Part model, mm, in its own coordinate system. A direction names the side the tool comes from. Give positions to 0.01 mm unless a question says otherwise; leave off trailing zeros. Order: outer loops, then holes, each group sorted by start corner. A loop starts at its lowest first (then second) coordinate and runs counter-clockwise, first axis right, second up.
Autodesk Inventor part; units mm, degrees
ref_plane "YZ Plane" through (0, 0, 0) normal (1, 0, 0) x (0, 1, 0)
ref_plane "XZ Plane" through (0, 0, 0) normal (0, 1, 0) x (-1, 0, 0)
ref_plane "XY Plane" through (0, 0, 0) normal (0, 0, 1) x (1, 0, 0)
sketch "Sketch2" plane through (0, 0, 0) normal (0, 0, 1) x (1, 0, 0)
  circle A0 centre (138.7343, -109.7729) radius 5.25
  circle A1 centre (116.8119, -56.8475) radius 5.25
  circle A2 centre (26.4627, 2.4988) radius 5.25
  circle A3 centre (79.388, -19.4236) radius 5.25
  line L0 (116.6514, -65.861) -> (120.8614, -63.1603)
  arc A4 (120.8614, -63.1603) -> (112.4329, -50.7586) centre (116.8119, -56.8475) ccw
  line L1 (112.4329, -50.7586) -> (108.3722, -53.679)
  arc A5 (108.3722, -53.679) -> (82.5566, -27.8633) centre (0, -136.2355) ccw
  line L2 (82.5566, -27.8633) -> (85.4769, -23.8026)
  arc A6 (85.4769, -23.8026) -> (73.0752, -15.3741) centre (79.388, -19.4236) ccw
  line L3 (73.0752, -15.3741) -> (70.3746, -19.5842)
  arc A7 (70.3746, -19.5842) -> (32.7226, -3.9882) centre (0, -136.2355) ccw
  line L4 (32.7226, -3.9882) -> (33.7899, 0.8984)
  arc A8 (33.7899, 0.8984) -> (19.0608, 3.7079) centre (26.4627, 2.4988) ccw
  line L5 (19.0608, 3.7079) -> (18.2544, -1.2285)
  arc A9 (18.2544, -1.2285) -> (0, 0) centre (0, -136.2355) ccw
  line L6 (0, 0) -> (0, -2)
  arc A10 (134.2355, -136.2355) -> (0, -2) centre (0, -136.2355) ccw
  line L7 (134.2355, -136.2355) -> (136.2355, -136.2355)
  arc A11 (136.2355, -136.2355) -> (135.007, -117.9811) centre (0, -136.2355) ccw
  line L8 (135.007, -117.9811) -> (139.9434, -117.1747)
  arc A12 (139.9434, -117.1747) -> (137.1339, -102.4456) centre (138.7343, -109.7729) ccw
  line L9 (137.1339, -102.4456) -> (132.2473, -103.5129)
  arc A13 (132.2473, -103.5129) -> (116.6514, -65.861) centre (0, -136.2355) ccw
  arc A14 (18.2544, -1.2285) -> (-23.9798, -2.127) centre (0, -136.2355) ccw
  arc A15 (-27.0685, -2.7162) -> (-23.9798, -2.127) centre (-26.4627, 2.4988) ccw
  arc A16 (-27.0685, -2.7162) -> (-75.2721, -22.6828) centre (0, -136.2355) ccw
  arc A17 (-77.8727, -24.4502) -> (-75.2721, -22.6828) centre (-79.388, -19.4236) ccw
  arc A18 (-77.8727, -24.4502) -> (-111.7853, -58.3628) centre (0, -136.2355) ccw
  arc A19 (-113.5527, -60.9634) -> (-111.7853, -58.3628) centre (-116.8119, -56.8475) ccw
  arc A20 (-113.5527, -60.9634) -> (-133.5193, -109.1671) centre (0, -136.2355) ccw
  arc A21 (-134.1085, -112.2557) -> (-133.5193, -109.1671) centre (-138.7343, -109.7729) ccw
  arc A22 (-134.1085, -112.2557) -> (-136.2355, -136.2355) centre (0, -136.2355) ccw
  line L10 (-136.2355, -136.2355) -> (-134.2355, -136.2355)
  arc A23 (-133.4843, -122.0537) -> (-134.2355, -136.2355) centre (0, -136.2355) ccw
  arc A24 (-133.2582, -120.0666) -> (-133.4843, -122.0537) centre (0, -136.2355) ccw
  arc A25 (-124.3552, -85.689) -> (-133.2582, -120.0666) centre (0, -136.2355) ccw
  arc A26 (-123.5884, -83.8419) -> (-124.3552, -85.689) centre (0, -136.2355) ccw
  arc A27 (-90.6982, -37.2759) -> (-123.5884, -83.8419) centre (0, -136.2355) ccw
  arc A28 (-89.2138, -35.9356) -> (-90.6982, -37.2759) centre (0, -136.2355) ccw
  arc A29 (-24.5369, -4.2616) -> (-89.2138, -35.9356) centre (0, -136.2355) ccw
  line L11 (-24.5369, -4.2616) -> (-17.9914, -35.5817)
  arc A30 (-24.3732, -35.8597) -> (-17.9914, -35.5817) centre (-22.5679, -3.9107) ccw
  arc A31 (-24.3732, -35.8597) -> (-71.7399, -55.1686) centre (-13.0409, -131.4111) ccw
  line L12 (-71.7399, -55.1686) -> (-89.2138, -35.9356)
  line L13 (-89.2138, -35.9356) -> (-90.6982, -37.2759)
  line L14 (-90.6982, -37.2759) -> (-74.6321, -57.4663)
  arc A32 (-74.6321, -57.4663) -> (-103.6394, -92.1242) centre (2.2704, -151.2986) ccw
  line L15 (-103.6394, -92.1242) -> (-123.5884, -83.8419)
  line L16 (-123.5884, -83.8419) -> (-124.3552, -85.689)
  line L17 (-124.3552, -85.689) -> (-104.606, -93.8884)
  arc A33 (-104.606, -93.8884) -> (-115.4523, -121.9752) centre (2.2704, -151.2986) ccw
  line L18 (-115.4523, -121.9752) -> (-133.2582, -120.0666)
  line L19 (-133.2582, -120.0666) -> (-133.4843, -122.0537)
  line L20 (-133.4843, -122.0537) -> (-115.9197, -123.9199)
  arc A34 (-115.9197, -123.9199) -> (-118.1107, -136.2355) centre (2.2704, -151.2986) ccw
  line L21 (-118.1107, -136.2355) -> (-115.1005, -136.2355)
  arc A35 (-69.7224, -57.3892) -> (-115.1005, -136.2355) centre (4.4084, -152.5347) ccw
  arc A36 (-15.6263, -37.1945) -> (-69.7224, -57.3892) centre (-7.9541, -140.298) ccw
  arc A37 (-15.6263, -37.1945) -> (18.2544, -1.2285) centre (-20.5393, 1.3748) ccw
  circle A38 centre (26.4627, 2.4988) radius 7.5
  point P0 (19.0608, 3.7079)
  point P1 (22.5679, -3.9107)
extrude "Extrusion2" add sketch "Sketch2" along normal blind 30 contours A13 L9 A12 L8 A11 L7 A10 A38 L4 A7 L3 A6 L2 A5 L1 A4 L0 | A10 A38 A8
sketch "Sketch3" plane through (0, 0, 30) normal (0, 0, 1) x (1, 0, 0)
  line L0 (32.7226, -3.9882) -> (33.7899, 0.8984)
  arc A0 (33.7899, 0.8984) -> (22.5679, -3.9107) centre (26.4627, 2.4988) ccw
  arc A1 (134.2355, -136.2355) -> (22.5679, -3.9107) centre (0, -136.2355) ccw
  line L1 (134.2355, -136.2355) -> (136.2355, -136.2355)
  arc A2 (136.2355, -136.2355) -> (135.007, -117.9811) centre (0, -136.2355) ccw
  line L2 (135.007, -117.9811) -> (139.9434, -117.1747)
  arc A3 (139.9434, -117.1747) -> (137.1339, -102.4456) centre (138.7343, -109.7729) ccw
  line L3 (137.1339, -102.4456) -> (132.2473, -103.5129)
  arc A4 (132.2473, -103.5129) -> (116.6514, -65.861) centre (0, -136.2355) ccw
  line L4 (116.6514, -65.861) -> (120.8614, -63.1603)
  arc A5 (120.8614, -63.1603) -> (112.4329, -50.7586) centre (116.8119, -56.8475) ccw
  line L5 (112.4329, -50.7586) -> (108.3722, -53.679)
  arc A6 (108.3722, -53.679) -> (82.5566, -27.8633) centre (0, -136.2355) ccw
  line L6 (82.5566, -27.8633) -> (85.4769, -23.8026)
  arc A7 (85.4769, -23.8026) -> (73.0752, -15.3741) centre (79.388, -19.4236) ccw
  line L7 (73.0752, -15.3741) -> (70.3746, -19.5842)
  arc A8 (70.3746, -19.5842) -> (32.7226, -3.9882) centre (0, -136.2355) ccw
  circle A9 centre (26.4627, 2.4988) radius 5.25
  circle A10 centre (79.388, -19.4236) radius 5.25
  circle A11 centre (116.8119, -56.8475) radius 5.25
  circle A12 centre (138.7343, -109.7729) radius 5.25
  circle A13 centre (0, -136.2355) radius 136.2355
  point P0 (0, 0)
  point P1 (133.5193, -109.1671)
  point P2 (134.1085, -112.2557)
  point P3 (135.007, -117.9811)
  point P4 (111.7853, -58.3628)
  point P5 (113.5527, -60.9634)
  point P6 (116.6514, -65.861)
  point P7 (27.0685, -2.7162)
  point P8 (20.1131, -1.4929)
  point P9 (23.9798, -2.127)
  point P10 (75.2721, -22.6828)
  point P11 (77.8727, -24.4502)
  point P12 (82.5566, -27.8633)
extrude "Extrusion3" cut sketch "Sketch3" against normal blind 20 contours A13 A9 A0 L0 | L7 A7 L6 A13 A10 | A13 A12 L3 A3 L2 | L5 A5 L4 A13 A11
sketch "Sketch4" plane through (0, 0, 10) normal (0, 0, 1) x (1, 0, 0)
  line L0 (33.7899, 0.8984) -> (32.7226, -3.9882)
  arc A0 (33.7899, 0.8984) -> (20.1131, -1.4929) centre (26.4627, 2.4988) ccw
  arc A1 (23.9798, -2.127) -> (20.1131, -1.4929) centre (0, -136.2355) ccw
  arc A2 (27.0685, -2.7162) -> (23.9798, -2.127) centre (26.4627, 2.4988) ccw
  arc A3 (32.7226, -3.9882) -> (27.0685, -2.7162) centre (0, -136.2355) ccw
  point P0 (0, 0)
extrude "Extrusion4" add sketch "Sketch4" along normal blind 8
properties part number "HalfFilterwall3"
Item 1: Pull direction Y, two halves, no side cores. Call faces 4 (the face through (134.6, -115.2, 20.1)), 5 (the face through (112.942, -60.396, 8.123)), 6 (the face through (144, -108, 10)), 7 (the face through (101.734, -48.66, 14.79)): released by +Y, released by -Y, zero draft, split by the parting line, or undercut.
Item 2: Drill centre lines: probe 1 along X at (y, z) = (-18, 3.25); probe 2 along X at (y, z) = (-60, 7.5); probe 3 along X at (y, z) = (0, 6.5). Where is each one in solid material? Low to high.
Item 3: Band-saw the part on D-D on y = -88. List the corners of the cut face in (x, z).
Item 4: Band-saw the part on C-C on z = 4.25. List the corners of the cut face in (x, y).
Item 5: Band-saw the part on A-A on x = 80. List the corners of the cut face in (y, z).
Item 6: Which spindle directions (+Z, -Z, +X, -X, +Y, -Y) get a long thin tool onto all of the face, cutting with end or side? Do faces 1 (the face through (72.874, -21.129, 20.14)), 2 (the face through (133.49, -110, 8.12)), 3 (the face through (71.744, -17.45, 4.93)). Say none if no direction does.
Item 7: Drop flat-ended pins along their axis: P1, Ø9.5, axis at x = 116.81, y = -56.85, coming from the -Z side; P2, Ø5, axis at x = 54.5, z = 6, coming from the -Y side; P3, Ø6, axis at x = 54, z = 15.5, coming from the +Y side; P4, Ø4, axis at x = 37.5, z = 9, coming from the -Y side. Give the stop position or say it passes through.
Working result:
1. face 4: released by +Y
1. face 5: undercut
1. face 6: zero draft
1. face 7: released by -Y
2. probe 1: x = 63.56 to 67.68, 71.39 to 74.33, 84.44 to 86.75
2. probe 2: x = 110.49 to 112.61, 121.01 to 123.62
2. probe 3: x = 19.39 to 21.85, 31.08 to 33.59
3. outline: (125.27, 0) - (127.41, 0) - (127.41, 30) - (125.27, 30) - close
4. outline: (19.06, 3.71) arc R7.5 ccw to (22.57, -3.91) arc R134.24 cw to (134.24, -136.24) - (136.24, -136.24) arc R136.24 ccw to (135.01, -117.98) - (139.94, -117.17) arc R7.5 ccw (long way) to (137.13, -102.45) - (132.25, -103.51) arc R136.24 ccw to (116.65, -65.86) - (120.86, -63.16) arc R7.5 ccw (long way) to (112.43, -50.76) - (108.37, -53.68) arc R136.24 ccw to (82.56, -27.86) - (85.48, -23.8) arc R7.5 ccw (long way) to (73.08, -15.37) - (70.37, -19.58) arc R136.24 ccw to (32.72, -3.99) - (33.79, 0.9) arc R7.5 ccw (long way) to start; hole circle Ø10.5 at (26.46, 2.5); hole circle Ø10.5 at (79.39, -19.42); hole circle Ø10.5 at (116.81, -56.85); hole circle Ø10.5 at (138.73, -109.77)
5. outline: (-28.44, 0) - (-24.64, 0) - (-24.64, 10) - (-25.96, 10) - (-25.96, 30) - (-28.44, 30) - close; (-14.21, 0) - (-11.95, 0) - (-11.95, 10) - (-14.21, 10) - close
6. face 1: +Z, +X, +Y
6. face 2: +Z, -Z
6. face 3: +Z, -Z, +Y
7. P1: passes through
7. P2: stops at y = -14.7
7. P3: stops at y = -9.91
7. P4: stops at y = -7.94
